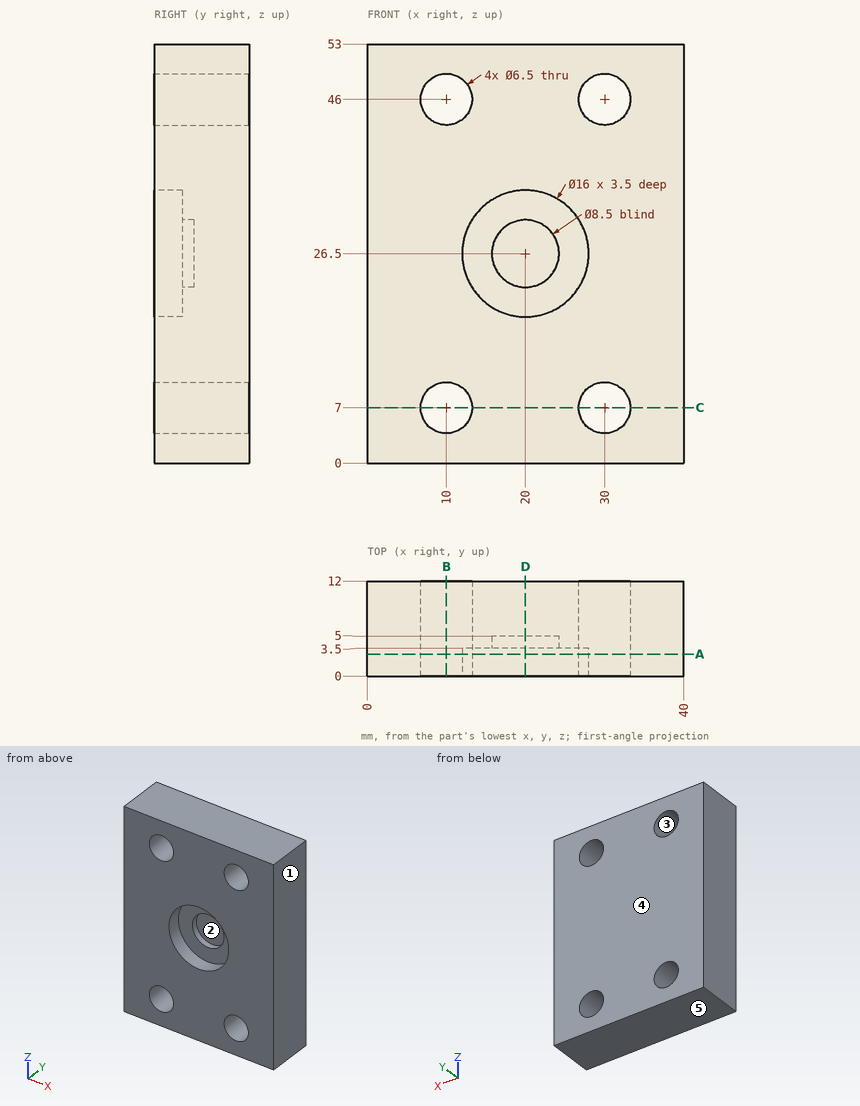
Geometry check sheet. Reference: drawing and pictorial views, mm from the part's lowest x, y, z. A direction names the side the tool comes from. Give positions to 0.01 mm unless a question says otherwise; leave off trailing zeros. Loops run counter-clockwise (first coordinate to the right, second up) from the corner with the lowest first, then second, coordinate; pieces in that order, holes last. Notation, with made-up numbers: (-32.75, 47) - (-26.75, 47) arc R24 cw to (-26.75, 80) - close; hole circle Ø11 at (64, -2). An arc over 180 degrees is marked (long way). Use CSV: the item, a comma, the result in double quotes. Start each with the question number.
Q1. Section check B-B, the plane x = 10. Record the cut outline in (y, z).
Q2. Section check D-D, the plane x = 20. Record the cut outline in (y, z).
Q3. Scan lines: probe 1 along X at (y, z) = (6.75, 46); probe 2 along Z at (x, y) = (10, 9.75); probe 3 along Z at (x, y) = (20, 4.05). Record each from-to range of solid material in increasing order. Write a range as from..to.
Q4. Section check C-C, the plane z = 7. Record the cut outline in (x, y).
Q5. Section check A-A, the plane y = 2.75. Record the cut outline in (x, z), and give its area (3 significant figures).
Q6. Release check for a two-part mould opening along Z. For the marked faces 3, 4 and 5 record: +Z half, -Z half, draft (parallel to the pull), parting line (faces both ways), or undercut.
Q7. Go/stop test with flat-tipped pins: pin 1 Ø5 at (x, z) = (24, 29.5) entering from -Y; pin 2 Ø5 at (x, z) = (30, 46) entering from -Y. Record where each tip stops, or that it passes through.
Q8. Access from +Z, -Z, +X, -X, +Y, -Y to the whole of each face (thin tool, end or side, straight path). Record for the marked faces 1 and 2.
Findings below:
1,outline,"(0, 0) - (12, 0) - (12, 3.75) - (0, 3.75) - close; (0, 10.25) - (12, 10.25) - (12, 42.75) - (0, 42.75) - close; (0, 49.25) - (12, 49.25) - (12, 53) - (0, 53) - close"
2,outline,"(0, 0) - (12, 0) - (12, 53) - (0, 53) - (0, 34.5) - (3.5, 34.5) - (3.5, 30.75) - (5, 30.75) - (5, 22.25) - (3.5, 22.25) - (3.5, 18.5) - (0, 18.5) - close"
3,probe 1,"x = 0..6.75, 13.25..26.75, 33.25..40"
3,probe 2,"z = 0..3.75, 10.25..42.75, 49.25..53"
3,probe 3,"z = 0..22.25, 30.75..53"
4,outline,"(0, 0) - (6.75, 0) - (6.75, 12) - (0, 12) - close; (13.25, 0) - (26.75, 0) - (26.75, 12) - (13.25, 12) - close; (33.25, 0) - (40, 0) - (40, 12) - (33.25, 12) - close"
5,outline,"(0, 0) - (40, 0) - (40, 53) - (0, 53) - close; hole circle Ø6.5 at (10, 7); hole circle Ø6.5 at (10, 46); hole circle Ø16 at (20, 26.5); hole circle Ø6.5 at (30, 7); hole circle Ø6.5 at (30, 46)"
5,area,"1,790 mm^2"
6,face 3,"undercut"
6,face 4,"draft"
6,face 5,"-Z half"
7,pin 1,"stops at y = 3.5"
7,pin 2,"passes through"
8,face 1,"+Z, -Z, +X, +Y, -Y"
8,face 2,"-Y"
